from build123d import *

# Parameters (mm, degrees)
SKETCH_1_W           = 61
SKETCH_1_H           = 32
EXTRUDE_1_DEPTH      = 6
SKETCH_2_R           = 10
CUT_EXTRUDE_13_DEPTH = 6
SKETCH_4_R           = 12
CUT_EXTRUDE_14_DEPTH = 5
SKETCH_5_W           = 12
SKETCH_5_H           = 15
CUT_EXTRUDE_16_DEPTH = 6
EXTRUDE_12_DEPTH     = 2
EXTRUDE_13_DEPTH     = 2
SKETCH_10_R          = 1.55
CUT_EXTRUDE_18_DEPTH = 15
SKETCH_11_R          = 1.55
CUT_EXTRUDE_19_DEPTH = 15


with BuildPart() as part:
    # Эскиз1 → Бобышка-Вытянуть1 (new body)
    with BuildSketch(Plane.XY):
        Rectangle(SKETCH_1_W, SKETCH_1_H)
    extrude(amount=EXTRUDE_1_DEPTH)

    # Эскиз2 → Вырез-Вытянуть13 (cut)
    with BuildSketch(Plane.XY.offset(6)):
        Circle(SKETCH_2_R)
    extrude(amount=-CUT_EXTRUDE_13_DEPTH, mode=Mode.SUBTRACT)

    # Эскиз4 → Вырез-Вытянуть14 (cut)
    with BuildSketch(Plane.XY.offset(6)):
        Circle(SKETCH_4_R)
    extrude(amount=-CUT_EXTRUDE_14_DEPTH, mode=Mode.SUBTRACT)

    # Эскиз5 → Вырез-Вытянуть16 (cut)
    with BuildSketch(Plane.XY.offset(6)):
        with Locations((21, 0)):
            Rectangle(SKETCH_5_W, SKETCH_5_H)
        with Locations((-21, 0)):
            Rectangle(SKETCH_5_W, SKETCH_5_H)
    extrude(amount=-CUT_EXTRUDE_16_DEPTH, mode=Mode.SUBTRACT)

    # Эскиз8 → Бобышка-Вытянуть12 (add)
    with BuildSketch(Plane.ZY.offset(30.5)):
        with BuildLine():
            Line((1.45, -1.5), (1.45, 1.4))
            ThreePointArc((1.45, 1.4), (2.9, 2.85), (4.35, 1.4))
            Line((4.35, 1.4), (4.35, -1.5))
            ThreePointArc((4.35, -1.5), (2.9, -2.95), (1.45, -1.5))
        make_face()
    extrude(amount=EXTRUDE_12_DEPTH)

    # Эскиз9 → Бобышка-Вытянуть13 (add)
    with BuildSketch(Plane(origin=(30.5, 0, 0), x_dir=(0, 0, -1), z_dir=(1, 0, 0))):
        with BuildLine():
            Line((-1.55, 1.45), (-1.55, -1.45))
            ThreePointArc((-1.55, -1.45), (-3, -2.9), (-4.45, -1.45))
            Line((-4.45, -1.45), (-4.45, 1.45))
            ThreePointArc((-4.45, 1.45), (-3, 2.9), (-1.55, 1.45))
        make_face()
    extrude(amount=EXTRUDE_13_DEPTH)

    # Эскиз10 → Вырез-Вытянуть18 (cut)
    with BuildSketch(Plane.ZY.offset(30.5)):
        with Locations(Location((3, 10, 0), (0, 0, 270))):  # turned: the seam where the file's is
            Circle(SKETCH_10_R)
        with Locations(Location((3, -11, 0), (0, 0, 270))):  # turned: the seam where the file's is
            Circle(SKETCH_10_R)
    extrude(amount=-CUT_EXTRUDE_18_DEPTH, mode=Mode.SUBTRACT)

    # Эскиз11 → Вырез-Вытянуть19 (cut)
    with BuildSketch(Plane(origin=(30.5, 0, 0), x_dir=(0, 0, -1), z_dir=(1, 0, 0))):
        with Locations(Location((-3, 11, 0), (0, 0, 90))):  # turned: the seam where the file's is
            Circle(SKETCH_11_R)
        with Locations(Location((-3, -11, 0), (0, 0, 270))):  # turned: the seam where the file's is
            Circle(SKETCH_11_R)
    extrude(amount=-CUT_EXTRUDE_19_DEPTH, mode=Mode.SUBTRACT)


solid = part.part
Verification items for the finished model (mm, model axes). A direction names the side the tool comes from. Coordinates: 2 decimals unless noted, no trailing zeros. Loops run counter-clockwise (first coordinate to the right, second up) from the corner with the lowest first, then second, coordinate; pieces in that order, holes last. Notation, with made-up numbers: (-20.75, 88.25) -> (16.25, 88.25) arc R13 cw to (16.25, 112.25) -> close; hole circle Ø2 at (76, 35.25). An arc over 180 degrees is marked (long way). Write each question's results on one line, items separated by ' | '.
Item 1: Section check B-B, the plane x = 0. Enter the section's corners in (y, z).
Found:
outline: (-16, 0) -> (-10, 0) -> (-10, 1) -> (-12, 1) -> (-12, 6) -> (-16, 6) -> close; (10, 0) -> (16, 0) -> (16, 6) -> (12, 6) -> (12, 1) -> (10, 1) -> close
Item 2: Mould release check, pull along Z, two halves, no side actions. Record for faces 5 (the face through (-5, 9, 1)), 6 (the face through (-27, 0, 3)), 7 (the face through (23.1, 9.77, 2.06)): +Z half, -Z half, draft (parallel to the pull), parting line (faces both ways), or undercut.
Found:
face 5: +Z half | face 6: draft | face 7: undercut
Item 3: Gauge pin test, flat ends, axial feed: pin 1 (2.5 mm diameter, centred on y = -11.5, z = 3, fed in from +X); pin 2 (5 mm diameter, centred on x = 1, y = -6.5, fed in from -Z); pin 3 (0.6 mm diameter, centred on x = -31.5, y = 0, fed in from -Z); pin 4 (1 mm diameter, centred on x = 31.5, y = 0, fed in from +Z). Record the tip position at first contact, or that the pin passes through.
Found:
pin 1: stops at x = 30.5 | pin 2: passes through | pin 3: stops at z = 1.45 | pin 4: stops at z = 4.45
Item 4: Material ranges on L1, parallel to Z at x = -22.25, y = 10; L2, parallel to Y at x = 0, z = 0.65; L3, parallel to Y at x = -15.5, z = 1.45, recorded low to high.
Found:
L1: z = 0 to 1.45, 4.55 to 6 | L2: y = -16 to -10, 10 to 16 | L3: y = -16 to -7.5, 7.5 to 16
Item 5: Section check D-D, the plane x = -6.5. Enter the section's corners in (y, z), plus the area to 3 significant figures.
Found:
outline: (-16, 0) -> (-7.6, 0) -> (-7.6, 1) -> (-10.09, 1) -> (-10.09, 6) -> (-16, 6) -> close; (7.6, 0) -> (16, 0) -> (16, 6) -> (10.09, 6) -> (10.09, 1) -> (7.6, 1) -> close | area: 75.9 mm2
Item 6: Section check C-C, the plane y = 0. Enter the section's corners in (x, z), plus the area to 3 significant figures.
Found:
outline: (-32.5, 1.45) -> (-30.5, 1.45) -> (-30.5, 0) -> (-27, 0) -> (-27, 6) -> (-30.5, 6) -> (-30.5, 4.35) -> (-32.5, 4.35) -> close; (-15, 0) -> (-10, 0) -> (-10, 1) -> (-12, 1) -> (-12, 6) -> (-15, 6) -> close; (10, 0) -> (15, 0) -> (15, 6) -> (12, 6) -> (12, 1) -> (10, 1) -> close; (27, 0) -> (30.5, 0) -> (30.5, 1.55) -> (32.5, 1.55) -> (32.5, 4.45) -> (30.5, 4.45) -> (30.5, 6) -> (27, 6) -> close | area: 93.6 mm2
Item 7: Tool access check on faces 1 (the face through (-23.1, -9.77, 2.06)), 2 (the face through (31.5, 2.9, 3)), 3 (the face through (-11.99, 0.53, 3.54)), 4 (the face through (-21, 7.5, 3)). Record the directions out of +Z, -Z, +X, -X, +Y, -Y that give a thin tool (end or side, any length) a straight path to the whole face; none if there is none.
Found:
face 1: -X | face 2: +X, +Y | face 3: +Z | face 4: +Z, -Z
Item 8: Section check A-A, the plane x = 22. Enter the section's corners in (y, z).
Found:
outline: (-16, 0) -> (-7.5, 0) -> (-7.5, 6) -> (-16, 6) -> close; (7.5, 0) -> (16, 0) -> (16, 6) -> (7.5, 6) -> close; hole circle Ø3.1 at (-11, 3); hole circle Ø3.1 at (11, 3)
